Source: CAD feature listing. Evaluate the final solid. Frame: model axes, mm. Face numbers are marked on the shaded views. Give positions to 0.01 mm unless a question says otherwise; leave off trailing zeros. Write each loop counter-clockwise with the first axis right and the second up, starting at its lowest first coordinate (ties: lowest second). Pieces come first, ordered by that corner, then holes.
```python
from build123d import *

# Parameters (mm, degrees)
SKETCH1_R                   = 2.25
BASEBOSS_EXTRUDE1_DEPTH     = 1.42
WINGBOSS_EXTRUDE2_DEPTH     = 28.58
FRONTCHAMFER1_SIZE          = 21.26
BACKCHAMFER3_SIZE           = 13
BACKCORNERFILLET1_R         = 2
RIGHTWINGCUT_EXTRUDE1_DEPTH = 117.224315421
LEFTWINGCUT_EXTRUDE2_DEPTH  = 114.155281671
OUTSIDEWINGFILLET2_R        = 1.35
INSIDEWINGFILLET3_R         = 1.35
INSIDECUTOUTFILLET4_R       = 1.35


with BuildPart() as part:
    # Sketch1 → BaseBoss-Extrude1 (new body)
    with BuildSketch(Plane(origin=(0, 0, 0), x_dir=(1, 0, 0), z_dir=(0, 1, 0))):
        Polygon((0, 0), (46, 0), (90.65, 44.65), (-44.65, 44.65), align=None)
        with Locations(Location((23, 39.4, 0), (0, 0, 90))):
            Circle(SKETCH1_R, mode=Mode.SUBTRACT)
        with Locations(Location((23, 5.25, 0), (0, 0, 90))):
            Circle(SKETCH1_R, mode=Mode.SUBTRACT)
        with Locations(Location((39.780728009, 5.25, 0), (0, 0, 90))):
            Circle(SKETCH1_R, mode=Mode.SUBTRACT)
        with Locations(Location((6.219271991, 5.25, 0), (0, 0, 90))):
            Circle(SKETCH1_R, mode=Mode.SUBTRACT)
        Polygon((-16.980980541, 25.268272016), (-2.962708524, 11.25), (48.962708524, 11.25), (62.980980541, 25.268272016), (54.849252557, 33.4), (-8.849252557, 33.4), align=None, mode=Mode.SUBTRACT)
    extrude(amount=BASEBOSS_EXTRUDE1_DEPTH)

    # Sketch2 → WingBoss-Extrude2 (add)
    with BuildSketch(Plane(origin=(0, 1.42, 0), x_dir=(1, 0, 0), z_dir=(0, 1, 0))):
        Polygon((-52.641816741, 54.65), (1.004091629, 1.004091629), (0, 0), (-53.645908371, 53.645908371), align=None)
        Polygon((44.995908371, 1.004091629), (46, 0), (99.645908371, 53.645908371), (98.641816741, 54.65), align=None)
    extrude(amount=WINGBOSS_EXTRUDE2_DEPTH)

    # FrontChamfer1
    frontchamfer1_edges = [part.edges().sort_by_distance(p)[0] for p in [
        (45.497954185, 30, -0.502045815),
        (0.502045815, 30, -0.502045815),
    ]]
    chamfer(frontchamfer1_edges, length=FRONTCHAMFER1_SIZE)

    # BackChamfer3
    backchamfer3_edges = [part.edges().sort_by_distance(p)[0] for p in [
        (-53.143862556, 1.42, -54.147954185),
        (99.143862556, 1.42, -54.147954185),
    ]]
    chamfer(backchamfer3_edges, length=BACKCHAMFER3_SIZE)

    # BackCornerFillet1
    backcornerfillet1_edges = [part.edges().sort_by_distance(p)[0] for p in [
        (99.143862556, 30, -54.147954185),
        (-53.143862556, 30, -54.147954185),
    ]]
    fillet(backcornerfillet1_edges, radius=BACKCORNERFILLET1_R)

    # Sketch3 → RightWingCut-Extrude1 (cut, through all)
    with BuildSketch(Plane(origin=(1.004091629, 0, -1.004091629), x_dir=(-0.7071067811865479, 0, -0.7071067811865471), z_dir=(0.7071067811865471, 0, -0.7071067811865479))):
        with BuildLine():
            Line((64.870634402, 15.004344422), (67.473088065, 15.004351159))
            ThreePointArc((67.473088065, 15.004351159), (69.47743754, 13.002598346), (67.478284754, 10.995655578))
            Line((67.478284754, 10.995655578), (64.870634402, 10.995655578))
            ThreePointArc((64.870634402, 10.995655578), (59.348088065, 13), (64.870634402, 15.004344422))
        make_face()
        with BuildLine():
            Line((34.870634402, 15.004344422), (37.473088065, 15))
            ThreePointArc((37.473088065, 15), (39.473088065, 13), (37.473088065, 11))
            Line((37.473088065, 11), (34.870634402, 10.995655578))
            ThreePointArc((34.870634402, 10.995655578), (29.348088065, 13), (34.870634402, 15.004344422))
        make_face()
    extrude(amount=-RIGHTWINGCUT_EXTRUDE1_DEPTH, mode=Mode.SUBTRACT)

    # Sketch4 → LeftWingCut-Extrude2 (cut, through all)
    with BuildSketch(Plane(origin=(21.995908371, 0, 21.995908371), x_dir=(-0.7071067811865476, 0, 0.7071067811865476), z_dir=(-0.7071067811865476, 0, -0.7071067811865476))):
        with BuildLine():
            Line((-97.397545502, 10.995654579), (-100.005197879, 10.995654579))
            ThreePointArc((-100.005197879, 10.995654579), (-102.004350476, 13.002598942), (-100, 15.004352161))
            Line((-100, 15.004352161), (-97.397545502, 15.004345421))
            ThreePointArc((-97.397545502, 15.004345421), (-91.875, 13), (-97.397545502, 10.995654579))
        make_face()
        with BuildLine():
            Line((-67.397545502, 10.995654579), (-70, 11))
            ThreePointArc((-70, 11), (-72, 13), (-70, 15))
            Line((-70, 15), (-67.397545502, 15.004345421))
            ThreePointArc((-67.397545502, 15.004345421), (-61.875, 13), (-67.397545502, 10.995654579))
        make_face()
    extrude(amount=-LEFTWINGCUT_EXTRUDE2_DEPTH, mode=Mode.SUBTRACT)

    # outsideWingFillet2
    outsidewingfillet2_edges = [part.edges().sort_by_distance(p)[0] for p in [
        (68.325, 0, -22.325),
        (-22.325, 0, -22.325),
    ]]
    fillet(outsidewingfillet2_edges, radius=OUTSIDEWINGFILLET2_R)

    # InsideWingFillet3
    insidewingfillet3_edges = [part.edges().sort_by_distance(p)[0] for p in [
        (66.818862556, 1.42, -22.827045815),
        (-20.818862556, 1.42, -22.827045815),
    ]]
    fillet(insidewingfillet3_edges, radius=INSIDEWINGFILLET3_R)

    # InsideCutoutFillet4
    insidecutoutfillet4_edges = [part.edges().sort_by_distance(p)[0] for p in [
        (48.962708524, 0.71, -11.25),
        (62.980980541, 0.71, -25.268272016),
        (54.849252557, 0.71, -33.4),
        (-8.849252557, 0.71, -33.4),
        (-16.980980541, 0.71, -25.268272016),
        (-2.962708524, 0.71, -11.25),
    ]]
    fillet(insidecutoutfillet4_edges, radius=INSIDECUTOUTFILLET4_R)


solid = part.part
```
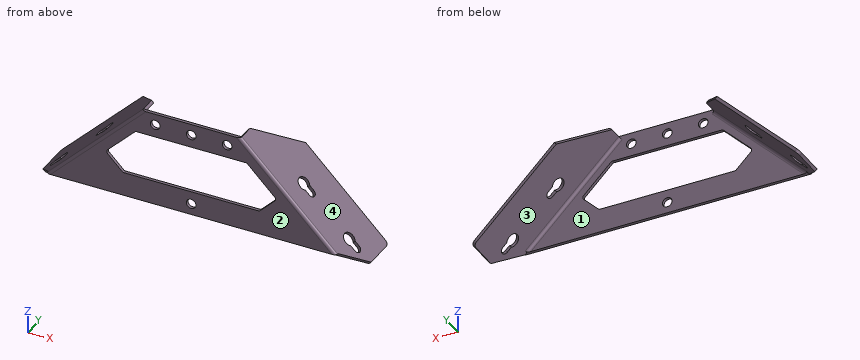
1. Section query A-A (x = 27). Return loops of the section in (y, z).
2. Section query B-B (y = 21). Return loops of the section in (x, z).
3. Section query C-C (z = -5.25). Give the number of separate pieces and of enclosed holes in the cut face, plus the area to 3 significant figures.
4. Pull-direction query (X, two-part tool) for the marked faces 1, 2, 3 and 4; classes: pulls with the +X half, pulls with the -X half, needs draft (parallel to the pull), parting line crosses it, or undercut.
5. Line query: probe 1 along Z at (x, y) = (23, 0.9); probe 2 along Y at (x, z) = (9, -5); probe 3 along X at (y, z) = (0.3, -5.25). Output: solid intervals per line, ascending.
6. Pin query (flat end, axial travel): P1, Ø2, axis at y = 12, z = -42.5, coming from the +X side; P2, Ø2, axis at x = 72, y = 23.5, coming from the +Z side; P3, Ø1.4, axis at x = 92, z = -46.5, coming from the -Y side; P4, Ø4, axis at x = 6.22, z = -5.25, coming from the +Y side. Return the tip coordinate at first contact, or that it passes through.
The answers:
1. outline: (0, -44.65) - (1.42, -44.65) - (1.42, -33.4) - (0, -33.4) - close; (0, -11.25) - (1.42, -11.25) - (1.42, 0) - (0, 0) - close
2. outline: (-53.65, -53.65) - (-52.64, -54.65) - (-7.67, -9.67) - (-8.67, -8.67) - close; (53.67, -9.67) - (98.64, -54.65) - (99.65, -53.65) - (54.67, -8.67) - close
3. separate pieces: 4
3. enclosed holes: 0
3. area: 117 mm2
4. face 1: undercut
4. face 2: needs draft
4. face 3: undercut
4. face 4: pulls with the +X half
5. probe 1: z = -44.65 to -41.65, -37.15 to -33.4, -11.25 to -7.5, -3 to 0
5. probe 2: y = 0 to 1.42
5. probe 3: x = -4.54 to 3.97, 8.47 to 20.75, 25.25 to 37.53, 42.03 to 50.54
6. P1: stops at x = 88.48
6. P2: stops at z = -25
6. P3: stops at y = 3.26
6. P4: passes through
